Solid Edge part; units mm, degrees
sketch "Sketch1" plane through (0, 0, 0) normal (0, -1, 0) x (1, 0, 0)
  line L0 (-16.825, -20) -> (-4.05, -20)
  line L1 (-4.05, -20) -> (-4.05, -15.5)
  line L2 (-4.05, -15.5) -> (-12.318, -15.5)
  line L3 (-12.318, -15.5) -> (-4.018, -7.2)
  line L4 (-4.018, -7.2) -> (4.018, -7.2)
  line L5 (4.018, -7.2) -> (12.318, -15.5)
  line L6 (12.318, -15.5) -> (4.05, -15.5)
  line L7 (4.05, -15.5) -> (4.05, -20)
  line L8 (4.05, -20) -> (16.825, -20)
  arc A0 (20, -16.825) -> (16.825, -20) centre (16.825, -16.825) cw
  line L9 (20, -16.825) -> (20, -4.0502)
  line L10 (20, -4.0502) -> (15.5, -4.0502)
  line L11 (15.5, -4.0502) -> (15.5, -12.318)
  line L12 (15.5, -12.318) -> (7.2, -4.018)
  line L13 (7.2, -4.018) -> (7.2, 4.018)
  line L14 (7.2, 4.018) -> (15.5, 12.318)
  line L15 (15.5, 12.318) -> (15.5, 4.0498)
  line L16 (15.5, 4.0498) -> (20, 4.0498)
  line L17 (20, 4.0498) -> (20, 16.825)
  arc A1 (16.825, 20) -> (20, 16.825) centre (16.825, 16.825) cw
  line L18 (16.825, 20) -> (4.05, 20)
  line L19 (4.05, 20) -> (4.05, 15.5)
  line L20 (4.05, 15.5) -> (12.318, 15.5)
  line L21 (12.318, 15.5) -> (4.018, 7.2)
  line L22 (4.018, 7.2) -> (-4.018, 7.2)
  line L23 (-4.018, 7.2) -> (-12.318, 15.5)
  line L24 (-12.318, 15.5) -> (-4.05, 15.5)
  line L25 (-4.05, 15.5) -> (-4.05, 20)
  line L26 (-4.05, 20) -> (-16.825, 20)
  arc A2 (-20, 16.825) -> (-16.825, 20) centre (-16.825, 16.825) cw
  line L27 (-20, 16.825) -> (-20, 4.05)
  line L28 (-20, 4.05) -> (-15.5, 4.05)
  line L29 (-15.5, 4.05) -> (-15.5, 12.318)
  line L30 (-15.5, 12.318) -> (-7.2, 4.018)
  line L31 (-7.2, 4.018) -> (-7.2, -4.018)
  line L32 (-7.2, -4.018) -> (-15.5, -12.318)
  line L33 (-15.5, -12.318) -> (-15.5, -4.05)
  line L34 (-15.5, -4.05) -> (-20, -4.05)
  line L35 (-20, -4.05) -> (-20, -16.825)
  arc A3 (-16.825, -20) -> (-20, -16.825) centre (-16.825, -16.825) cw
  circle A4 centre (0.1887, 0) radius 3
extrude "Protrusion1" add sketch "Sketch1" against normal blind 31.75
Can you work these out from the model? Positions are in its coordinate system, mm. A direction names the side the tool comes from. Round coordinates to 2 decimals unless told otherwise and drop trailing zeros. Loops run counter-clockwise (first coordinate to the right, second up) from the corner with the lowest first, then second, coordinate; pieces in that order, holes last. Notation, with made-up numbers: M -35,52.5 L -12,52.5 A13 ccw -12,63.5 Z; hole C 77.25,-39 d1. An arc over 180 degrees is marked long. Answer as a JSON object with one key per item and string values. Group by question number.
Q1. Imagine slicing it at A-A, the plane z = 0. Please give me the cut outline in (x, y).
Q2. Will these pins go through, and if not, where does the flat tip stop? pin 1 (3.5 mm diameter, centred on x = -19, y = 13.5, fed in from -Z); pin 2 (1.3 mm diameter, centred on x = 18, y = 10.5, fed in from +Z).
Q3. We'd pull the mould along Z, two halves only. Please class faces 1 (the flat face through (-4.05, 16, -18)), 2 (the flat face through (11, 16, 20)), 3 (the flat face through (8, 16, -15.5)): +Z half, -Z half, draft (parallel to the pull), parting line (faces both ways), or undercut.
Q4. On a 3-axis mill with a long thin cutter (end or side, diameter ignored), from which of +Z, -Z, +X, -X, +Y, -Y can I reach the whole of each face in a straight line? I mean faces 4 (the flat face through (-15.5, 16, 8)), 5 (the flat face through (-18, 16, 4.05)), 6 (the flat face through (18, 16, -4.05)), 7 (the flat face through (-4.05, 16, 18)). Say none if no direction works.
Q5. Imagine slicing it at C-C, the plane x = -6.5. Please give me the cut outline in (y, z).
Q6. Please list where these lines run through material, in increasing order: L1, parallel to Z at x = -7, y = 13; L2, parallel to Z at x = -6.5, y = 17.5; L3, parallel to X at y = 7.5, z = 5.5.
Q7. Imagine slicing it at B-B, the plane x = 13.5. Please give me the cut outline in (y, z).
Findings:
{
 "1": {"outline": "M -7.2,0 L -2.81,0 L -2.81,31.75 L -7.2,31.75 Z; M 3.19,0 L 7.2,0 L 7.2,31.75 L 3.19,31.75 Z"},
 "2": {"pin 1": "stops at z = -19.97", "pin 2": "stops at z = 19.96"},
 "3": {"face 1": "draft", "face 2": "+Z half", "face 3": "undercut"},
 "4": {"face 4": "+Y, -Y", "face 5": "-X, +Y, -Y", "face 6": "+X, +Y, -Y", "face 7": "+Z, +Y, -Y"},
 "5": {"outline": "M 0,-20 L 31.75,-20 L 31.75,-15.5 L 0,-15.5 Z; M 0,-9.68 L 31.75,-9.68 L 31.75,9.68 L 0,9.68 Z; M 0,15.5 L 31.75,15.5 L 31.75,20 L 0,20 Z"},
 "6": {"L1": "z = -20 to -15.5, -10.18 to 10.18, 15.5 to 20", "L2": "z = -20 to -15.5, -9.68 to 9.68, 15.5 to 20", "L3": "x = -20 to -15.5, -8.68 to 8.68, 15.5 to 20"},
 "7": {"outline": "M 0,-20 L 31.75,-20 L 31.75,-10.32 L 0,-10.32 Z; M 0,10.32 L 31.75,10.32 L 31.75,20 L 0,20 Z"}
}
